```python
from build123d import *

# Parameters (mm, degrees)
SKETCH2_W             = 130
SKETCH2_H             = 130
BOSS_EXTRUDE2_DEPTH   = 37.5
SKETCH3_W             = 80
SKETCH3_H             = 120
CUT_EXTRUDE1_DEPTH    = 67.5
SKETCH15_W            = 81.593666544
SKETCH15_H            = 171.523851769
CUT_EXTRUDE9_DEPTH    = 119.638105177
SKETCH5_W             = 12.5
SKETCH5_H             = 75
BOSS_EXTRUDE4_DEPTH   = 20
BOSS_EXTRUDE4_2_DEPTH = 20
SKETCH7_R             = 6
CUT_EXTRUDE10_DEPTH   = 20
BOSS_EXTRUDE7_DEPTH   = 5
SKETCH17_W            = 24
SKETCH17_H            = 37
CUT_EXTRUDE11_DEPTH   = 5
SKETCH18_R            = 5
BOSS_EXTRUDE8_DEPTH   = 10
LPATTERN2_COUNT       = 2
LPATTERN2_PITCH       = 55
CUT_EXTRUDE12_REACH   = 152.359
SKETCH20_R            = 25
SKETCH21_R            = 15
CUT_EXTRUDE13_DEPTH   = 10
BOSS_EXTRUDE9_DEPTH   = 80
SKETCH23_W            = 10
SKETCH23_H            = 7.5
BOSS_EXTRUDE10_DEPTH  = 80


with BuildPart() as part:
    # Sketch2 → Boss-Extrude2 (new, symmetric)
    with BuildSketch(Plane(origin=(0, 0, 0), x_dir=(1, 0, 0), z_dir=(0, 1, 0))):
        Rectangle(SKETCH2_W, SKETCH2_H)
    extrude(amount=BOSS_EXTRUDE2_DEPTH, both=True)

    # Sketch3 → Cut-Extrude1 (cut)
    with BuildSketch(Plane(origin=(0, 37.5, 0), x_dir=(1, 0, 0), z_dir=(0, 1, 0))):
        with Locations((25, 0)):
            Rectangle(SKETCH3_W, SKETCH3_H)
    extrude(amount=-CUT_EXTRUDE1_DEPTH, mode=Mode.SUBTRACT)

    # Sketch15 → Cut-Extrude9 (cut, through all)
    with BuildSketch(Plane(origin=(0, 37.5, 0), x_dir=(1, 0, 0), z_dir=(0, 1, 0))):
        with Locations((-65.796833272, -4.787594099)):
            Rectangle(SKETCH15_W, SKETCH15_H)
    extrude(amount=-CUT_EXTRUDE9_DEPTH, mode=Mode.SUBTRACT)


with BuildPart() as body_2:
    # Sketch5 → Boss-Extrude4 (new body)
    with BuildSketch(Plane(origin=(65, 0, 0), x_dir=(0, 0, -1), z_dir=(1, 0, 0))):
        with Locations((-71.25, 0)):
            Rectangle(SKETCH5_W, SKETCH5_H)
    extrude(amount=-BOSS_EXTRUDE4_DEPTH)


with BuildPart() as body_3:
    # Sketch5 → Boss-Extrude4 2 (new body)
    with BuildSketch(Plane(origin=(65, 0, 0), x_dir=(0, 0, -1), z_dir=(1, 0, 0))):
        with Locations((71.25, 0)):
            Rectangle(SKETCH5_W, SKETCH5_H)
    extrude(amount=-BOSS_EXTRUDE4_2_DEPTH)


with BuildPart() as cut_extrude10_tool:
    # Sketch7 → Cut-Extrude10 (new body)
    with BuildSketch(Plane(origin=(65, 0, 0), x_dir=(0, 0, -1), z_dir=(1, 0, 0))):
        with Locations((-67.475, 0)):
            Circle(SKETCH7_R)
        with Locations((67.475, 0)):
            Circle(SKETCH7_R)
    extrude(amount=-CUT_EXTRUDE10_DEPTH)


with BuildPart() as part_1:
    add(part.part)

    # Cut-Extrude10: cut by cut_extrude10_tool
    add(cut_extrude10_tool.part, mode=Mode.SUBTRACT)



with BuildPart() as body_2_1:
    add(body_2.part)

    # Cut-Extrude10: cut by cut_extrude10_tool
    add(cut_extrude10_tool.part, mode=Mode.SUBTRACT)


with BuildPart() as body_3_1:
    add(body_3.part)

    # Cut-Extrude10: cut by cut_extrude10_tool
    add(cut_extrude10_tool.part, mode=Mode.SUBTRACT)


with BuildPart() as part_2:
    add(part_1.part)

    add(body_2_1.part)  # Boss-Extrude7 merges body 2

    add(body_3_1.part)  # Boss-Extrude7 merges body 3
    # Sketch16 → Boss-Extrude7 (add)
    with BuildSketch(Plane(origin=(0, 37.5, 0), x_dir=(1, 0, 0), z_dir=(0, 1, 0))):
        Polygon((-25, 65), (-25, -65), (45, -65), (45, -77.5), (65, -77.5), (65, 77.5), (45, 77.5), (45, 65), align=None)
    extrude(amount=BOSS_EXTRUDE7_DEPTH)

    # Sketch17 → Cut-Extrude11 (cut)
    with BuildSketch(Plane.XY.offset(65)):
        with Locations((2, 6)):
            Rectangle(SKETCH17_W, SKETCH17_H)
    extrude(amount=-CUT_EXTRUDE11_DEPTH, mode=Mode.SUBTRACT)

    # Sketch18 → Boss-Extrude8 (add)
    # profile 1 of 2: a face of its own
    with BuildSketch(Plane.ZY.offset(25)):
        with BuildLine():
            Line((45, 42.5), (45, 60))
            ThreePointArc((45, 60), (58.75, 73.75), (72.5, 60))
            Line((72.5, 60), (72.5, 42.5))
            Line((72.5, 42.5), (45, 42.5))
        make_face()
        with Locations((58.75, 60)):
            Circle(SKETCH18_R, mode=Mode.SUBTRACT)
    # profile 2 of 2: a face of its own
    with BuildSketch(Plane.ZY.offset(25)):
        with BuildLine():
            Line((72.5, -37.5), (45, -37.5))
            Line((45, -37.5), (45, -55))
            ThreePointArc((45, -55), (58.75, -68.75), (72.5, -55))
            Line((72.5, -55), (72.5, -37.5))
        make_face()
        with Locations(Location((58.75, -55, 0), (0, 0, 180))):
            Circle(SKETCH18_R, mode=Mode.SUBTRACT)
    boss_extrude8 = extrude(amount=-BOSS_EXTRUDE8_DEPTH)

    # LPattern2: Boss-Extrude8 ×2
    with Locations(*[(0, 0, -i * LPATTERN2_PITCH) for i in range(1, LPATTERN2_COUNT)]):
        add(boss_extrude8)

    # Cut-Extrude12: up to this face of the body (flat: up to its plane)
    cut_extrude12_end = Plane(part_2.part.faces().sort_by_distance((23.113006397, -37.5, -1.026119403))[0])
    # Sketch20 → Cut-Extrude12 (cut, up to the picked face)
    with BuildSketch(Plane(origin=(0, 42.5, 0), x_dir=(1, 0, 0), z_dir=(0, 1, 0)), mode=Mode.PRIVATE) as cut_extrude12_sk1:
        with Locations(Location((15, 0, 0), (0, 0, 90))):
            Circle(SKETCH20_R)
    cut_extrude12_tool1 = split(extrude(cut_extrude12_sk1.sketch, amount=-CUT_EXTRUDE12_REACH, mode=Mode.PRIVATE), bisect_by=cut_extrude12_end, keep=Keep.BOTH, mode=Mode.PRIVATE)
    add(cut_extrude12_tool1.solids().sort_by(Axis((15, 42.5, 0), (0, -1, 0)))[0], mode=Mode.SUBTRACT)

    # Sketch21 → Cut-Extrude13 (cut)
    with BuildSketch(Plane.ZY.offset(25)):
        with Locations((30, 2.5)):
            Circle(SKETCH21_R)
        with Locations((-30, 2.5)):
            Circle(SKETCH21_R)
    extrude(amount=-CUT_EXTRUDE13_DEPTH, mode=Mode.SUBTRACT)

    # Sketch22 → Boss-Extrude9 (add)
    with BuildSketch(Plane(origin=(0, 42.5, 0), x_dir=(1, 0, 0), z_dir=(0, 1, 0))):
        Polygon((45, -65), (45, -77.5), (25, -65), align=None)
        Polygon((45, 77.5), (45, 65), (25, 65), align=None)
    extrude(amount=-BOSS_EXTRUDE9_DEPTH)

    # Sketch23 → Boss-Extrude10 (add)
    with BuildSketch(Plane(origin=(0, 42.5, 0), x_dir=(-1, 0, 0), z_dir=(0, -1, 0))):
        with Locations((20, -68.75)):
            Rectangle(SKETCH23_W, SKETCH23_H)
    extrude(amount=BOSS_EXTRUDE10_DEPTH)


solid = part_2.part
```
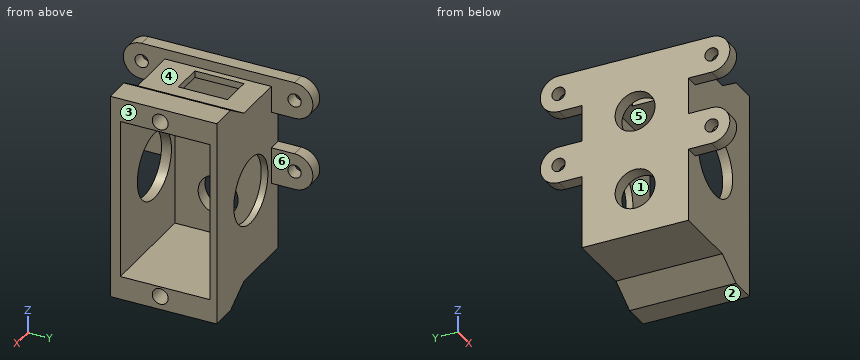
Here's how the part is built. I have some questions about the finished solid (model axes, mm). Face numbers are marked on the shaded views. A direction names the side the tool comes from. Coordinates: 2 decimals unless noted, no trailing zeros. Write each loop counter-clockwise with the first axis right and the second up, starting at its lowest first coordinate (ties: lowest second). Pieces come first, ordered by that corner, then holes. Notation, with made-up numbers: (-34.75, 26.5) -> (-3.75, 26.5) arc R23 cw to (-3.75, 48.5) -> close; hole circle Ø8 at (13, -12). An arc over 180 degrees is marked (long way). Use a Markdown table: item, result. Add a question column.
(1) Please list where these lines run through material, in increasing order: line 1 (Y direction, x = 52, z = 52.5); line 2 (X direction, y = 23, z = 63.5); line 3 (Z direction, x = -11, y = -10).
(2) If we section it at B-B, the plane y = 45.5: Write out the boundary of the cut face in (x, z).
(3) If we section it at A-A, the plane z = -30: Write out the boundary of the cut face in (x, y).
(4) If we section it at C-C, the plane y = 8: Write out the boundary of the cut face in (x, z).
(5) We'd pull the mould along Z, two halves only. Please class the marked faces 1, 2 and 3: +Z half, -Z half, draft (parallel to the pull), parting line (faces both ways), or undercut.
(6) If we section it at D-D, the plane y = -33: Write out the boundary of the cut face in (x, z), and give its area (3 significant figures).
(7) I'm going to push flat-ended pins straight in: P1, Ø24, axis at x = 20, z = 9.5, coming from the -Y side; P2, Ø1.5, axis at x = 8.5, y = 18, coming from the +Z side; P3, Ø8, axis at y = 13.5, z = 55.5, coming from the +X side; P4, Ø8, axis at x = -19, y = -48, coming from the +Z side. Where does each tip first touch, or does it pass through?
(8) For the marked faces 4, 5 and 6, which set-ups out of +Z, -Z, +X, -X, +Y, -Y let a thin tool reach every point of the face, with its end or its side?
Outcome:
| question | item | result |
|---|---|---|
| 1 | line 1 | y = -37.5 to -30, 37.5 to 42.5 |
| 1 | line 2 | x = -25 to -10, 14 to 65 |
| 1 | line 3 | z = -65 to -60, 60 to 65 |
| 2 | outline | (-25, -10) -> (-15, -10) -> (-15, 17.5) -> (-25, 17.5) -> close; (-25, 45) -> (-15, 45) -> (-15, 72.5) -> (-25, 72.5) -> close |
| 3 | outline | (-25, -37.5) -> (65, -37.5) -> (65, -30) -> (-15, -30) -> (-15, -12.5) -> (-25, -12.5) -> close; (-25, 17.5) -> (-15, 17.5) -> (-15, 37.5) -> (65, 37.5) -> (65, 42.5) -> (-25, 42.5) -> close |
| 4 | outline | (-25, -65) -> (25, -65) -> (45, -77.5) -> (65, -77.5) -> (65, -60) -> (-15, -60) -> (-15, -43.96) -> (-25, -43.96) -> close; (-25, -16.04) -> (-15, -16.04) -> (-15, 16.04) -> (-25, 16.04) -> close; (-25, 43.96) -> (-15, 43.96) -> (-15, 60) -> (-10, 60) -> (-10, 65) -> (-15, 65) -> (-15, 72.5) -> (-25, 72.5) -> close; (14, 60) -> (65, 60) -> (65, 77.5) -> (45, 77.5) -> (25, 65) -> (14, 65) -> close |
| 5 | face 1 | undercut |
| 5 | face 2 | -Z half |
| 5 | face 3 | draft |
| 6 | outline | (-25, -65) -> (25, -65) -> (45, -77.5) -> (65, -77.5) -> (65, 77.5) -> (45, 77.5) -> (25, 65) -> (-15, 65) -> (-15, 72.5) -> (-25, 72.5) -> close; hole circle Ø50 at (15, 0) |
| 6 | area | 10,600 mm^2 |
| 7 | P1 | passes through |
| 7 | P2 | stops at z = -60 |
| 7 | P3 | stops at x = -15 |
| 7 | P4 | stops at z = 72.5 |
| 8 | face 4 | +Z, +Y, -Y |
| 8 | face 5 | +X |
| 8 | face 6 | +Z, -Z, +X, +Y |
